Model file for the job. Use its own axes, mm. A direction names the side the tool comes from. Round coordinates to 2 decimals unless told otherwise and drop trailing zeros. Order: outer loops, then holes, each group sorted by start corner. A loop starts at its lowest first (then second) coordinate and runs counter-clockwise, first axis right, second up. Notation, with made-up numbers: (72, 79) - (85, 79) arc R25 ccw to (85, 113) - close; hole circle Ø6 at (76, -7). An arc over 180 degrees is marked (long way). Write item = value, one per line. Start each with the question number.
from build123d import *

# Parameters (mm, degrees)
F0_W     = 73.152
F0_H     = 5.744279672
F0_H_2   = 2.54
F1_DEPTH = 5.08
F0_W_2   = 6.35
F0_W_3   = 15.748
F0_H_3   = 3.1443536282
F2_DEPTH = 6.35
F0_H_4   = 65.5344708799
F0_H_5   = 9.6294713412
F3_DEPTH = 6.096


# Not quite as in the source:
# - a feature names something its author has since deleted; it is built from what else it names


with BuildPart() as f1:
    # F0 (on Front) → F1 (new body)
    with BuildSketch(Plane.XZ):
        Polygon((-44.2442491055, -63.1286278367), (-44.2442491055, -57.3843481647), (-44.2442491055, -40.2686278367), (-44.2442491055, -37.7286278367), (-44.2442491055, -32.8348538627), (-44.2442491055, -31.8823538627), (-44.2442491055, -30.9298538627), (-44.2442491055, -20.7698538627), (-44.2442491055, -19.8173538627), (-44.2442491055, -18.8648538627), (-44.2442491055, 9.1076644534), (-44.2442491055, 11.6476644534), (-44.2442491055, 15.1796680125), (-44.2442491055, 37.0476644534), (-44.2442491055, 44.6676644534), (-44.2442491055, 66.4113721633), (-50.5942491055, 66.4113721633), (-50.5942491055, -63.1286278367), align=None)
        with BuildLine():
            add(Edge.make_bspline(
                [(28.9077508945, 27.4595177274), (11.3712688144, 24.6047450509), (-13.4084815754, 35.2112312639), (-32.4729044871, 50.7994146886), (-44.2442491055, 44.6676644534)],
                knots=[0, 0, 0, 0, 0.5425588266, 1, 1, 1, 1], degree=3))
            Line((-44.2442491055, 44.6676644534), (-44.2442491055, 37.0476644534))
            add(Edge.make_bspline(
                [(28.9077508945, 19.8395177274), (11.5484302318, 18.9806314817), (-12.3449743232, 26.085082613), (-32.5652834278, 43.6948913941), (-44.2442491055, 37.0476644534)],
                knots=[0, 0, 0, 0, 0.5368571136, 1, 1, 1, 1], degree=3))
            Line((28.9077508945, 19.8395177274), (28.9077508945, 27.4595177274))
        make_face()
        Polygon((28.9077508945, -40.2686278367), (28.9077508945, -57.3843481647), (28.9077508945, -63.1286278367), (35.2577508945, -63.1286278367), (35.2577508945, 2.4058430432), (35.2577508945, 5.5501966713), (35.2577508945, 15.1796680125), (35.2577508945, 35.0404930887), (28.9077508945, 35.0404930887), (28.9077508945, 27.4595177274), (28.9077508945, 19.8395177274), (28.9077508945, 12.2195177274), (28.9077508945, 11.6476644534), (28.9077508945, 9.1076644534), (28.9077508945, -18.8648538627), (28.9077508945, -19.8173538627), (28.9077508945, -20.7698538627), (28.9077508945, -30.9298538627), (28.9077508945, -31.8823538627), (28.9077508945, -32.8348538627), (28.9077508945, -37.7286278367), align=None)
        with Locations((-7.6682491055, -60.2564880007)):
            Rectangle(F0_W, F0_H)
        with Locations((-7.6682491055, 10.3776644534)):
            Rectangle(F0_W, F0_H_2)
        with Locations((-7.6682491055, -38.9986278367)):
            Rectangle(F0_W, F0_H_2)
    extrude(amount=F1_DEPTH)

    # F0 (on Front) → F2 (join)
    with BuildSketch(Plane.XZ):
        with Locations((-47.4192491055, 67.6813721633)):
            Rectangle(F0_W_2, F0_H_2)
        with Locations((32.0827508945, 36.3104930887)):
            Rectangle(F0_W_2, F0_H_2)
        with Locations((43.1317508945, 3.9780198572)):
            Rectangle(F0_W_3, F0_H_3)
    extrude(amount=F2_DEPTH)

    # F0 (on Front) → F3 (join)
    with BuildSketch(Plane.XZ):
        with Locations((43.1317508945, -30.3613923968)):
            Rectangle(F0_W_3, F0_H_4)
        with Locations((43.1317508945, 10.3649323419)):
            Rectangle(F0_W_3, F0_H_5)
    extrude(amount=F3_DEPTH)


solid = f1.part
Item 1: Probe L1, parallel to X at y = -4, z = -5; L2, parallel to Z at x = -17.5, y = -2; L3, parallel to Z at x = -1.5, y = -1. List the from-to ranges inside material, lowest first.
Item 2: Mould opens along Z. For faces 4 (the face through (43, -3, 15.18)), 5 (the face through (35.258, -2, 26)), 6 (the face through (28.908, -3, 16)) say: +Z half, -Z half, draft (parallel to the pull), parting line (faces both ways), or undercut.
Item 3: Saw through at A-A, the plane z = -8.5. Give the cut face in (x, y), then the cut area to 3 significant figures.
Item 4: Saw through at C-C, the plane x = 4. Give the number of separate pieces and of enclosed holes in the cut face, then the cut area to 3 significant figures.
Item 5: Which spindle directions (+Z, -Z, +X, -X, +Y, -Y) get a long thin tool onto all of the face, cutting with end or side? Do faces 1 (the face through (28.908, -2, 33)), 2 (the face through (43, -6.096, 10)), 3 (the face through (-8, -3, 11.648)). Say none if no direction does.
Item 6: Saw through at B-B, the plane x = 44. Give the cut face in (y, z).
Item 7: Drop flat-ended pins along their axis: pin 1 (12 mm diameter, centred on x = 16.5, z = 26.5, fed in from -Y); pin 2 (2.5 mm diameter, centred on x = 0.5, y = -3, fed in from +Z); pin 3 (2 mm diameter, centred on x = -4.5, y = -4, fed in from +Z). Give the stop position or say it passes through.
Check sheet entries:
q1.L1 = -50.59 to -44.24, 28.91 to 51.01
q1.L2 = -63.13 to -57.38, -40.27 to -37.73, 9.11 to 11.65, 32.34 to 39.88
q1.L3 = -63.13 to -57.38, -40.27 to -37.73, 9.11 to 11.65, 24.12 to 31.14
q2.face_4 = +Z half
q2.face_5 = draft
q2.face_6 = undercut
q3.outline = (-50.59, -5.08) - (-44.24, -5.08) - (-44.24, 0) - (-50.59, 0) - close; (28.91, -5.08) - (35.26, -5.08) - (35.26, -6.1) - (51.01, -6.1) - (51.01, 0) - (28.91, 0) - close
q3.area = 161 mm2
q4.separate_pieces = 4
q4.enclosed_holes = 0
q4.area = 89.6 mm2
q5.face_1 = +Z, +Y, -Y
q5.face_2 = +Z, +X, -X, -Y
q5.face_3 = +Y, -Y
q6.outline = (-6.35, 2.41) - (-6.1, 2.41) - (-6.1, -63.13) - (0, -63.13) - (0, 15.18) - (-6.1, 15.18) - (-6.1, 5.55) - (-6.35, 5.55) - close
q7.pin_1 = -5.08
q7.pin_2 = 30.84
q7.pin_3 = 32.96
